from build123d import *

# Parameters (mm, degrees)
ESQUISSE1_R             = 1.7
BOSS_EXTRU_1_DEPTH      = 3
ENL_V_MAT_EXTRU_1_DEPTH = 25.197605652
CONG_1_R                = 3
CONG_2_R                = 3


with BuildPart() as part:
    # Esquisse1 → Boss.-Extru.1 (new body)
    with BuildSketch(Plane.XY):
        Polygon((12.594874651, 9.115771584), (-7.904447763, 6.416984589), (-2.628489378, 17.375533229), (16.571510622, 17.375533229), align=None)
        with Locations((8.467987162, 12.175533229)):
            Circle(ESQUISSE1_R, mode=Mode.SUBTRACT)
        with Locations((0.467987162, 12.175533229)):
            Circle(ESQUISSE1_R, mode=Mode.SUBTRACT)
    extrude(amount=BOSS_EXTRU_1_DEPTH)

    # Esquisse2 → Enlèv. mat.-Extru.1 (cut, through all)
    with BuildSketch(Plane.XY.offset(3)):
        with BuildLine():
            ThreePointArc((6.767987162, 12.175533229), (6.714089789, 12.99784824), (6.553319868, 13.806093213))
            ThreePointArc((6.553319868, 13.806093213), (7.755401396, 15.888159494), (9.837467677, 14.686077966))
            ThreePointArc((9.837467677, 14.686077966), (10.085002318, 13.441637293), (10.167987162, 12.175533229))
            ThreePointArc((10.167987162, 12.175533229), (8.467987162, 10.475533229), (6.767987162, 12.175533229))
        make_face()
    extrude(amount=-ENL_V_MAT_EXTRU_1_DEPTH, mode=Mode.SUBTRACT)

    # Congé1
    cong_1_edges = [part.edges().sort_by_distance(p)[0] for p in [
        (-2.628489378, 17.375533229, 1.5),
        (16.571510622, 17.375533229, 1.5),
        (12.594874651, 9.115771584, 1.5),
        (-7.904447763, 6.416984589, 1.5),
    ]]
    fillet(cong_1_edges, radius=CONG_1_R)

    # Congé2
    # the kernel refuses this fillet: 3 mm, written as the material it takes off along each edge
    with BuildSketch(Plane(origin=(-8.243247375, 17.375533229, 0), x_dir=(0, -1, 0), z_dir=(1, 0, 0))) as cong_2_piece_1:
        with BuildLine():
            CenterArc((CONG_2_R, -CONG_2_R), CONG_2_R, 90, 90)
            Line((0, -CONG_2_R), (0, 0))
            Line((0, 0), (CONG_2_R, 0))
        make_face()
    extrude(amount=27.54083508, mode=Mode.SUBTRACT)


solid = part.part
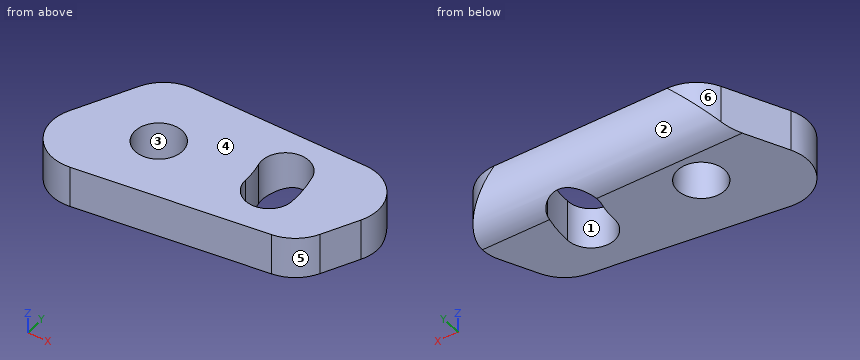
Work out the finished part from the listing and answer in its coordinate system (mm). Face numbers are marked on the shaded views. A direction names the side the tool comes from. Round coordinates to 2 decimals unless told otherwise and drop trailing zeros. Write each loop counter-clockwise with the first axis right and the second up, starting at its lowest first coordinate (ties: lowest second). Pieces come first, ordered by that corner, then holes. Notation, with made-up numbers: (72.25, 17) -> (92.25, 17) arc R22 ccw to (92.25, 38) -> close; hole circle Ø1 at (89, 6). An arc over 180 degrees is marked (long way). Write each question's results on one line, items separated by ' | '.
Item 1: A cutting plane is placed at A-A, the plane y = 15.25. Determine the outline of the cut face in (x, z), plus the area to 3 significant figures.
Result set:
outline: (-3.65, 0.13) -> (6.82, 0.13) -> (6.82, 3) -> (-3.65, 3) -> close; (9.57, 0.13) -> (14.67, 0.13) -> (14.67, 3) -> (9.57, 3) -> close | area: 44.7 mm^2
Item 2: Which of the six approach directions +Z, -Z, +X, -X, +Y, -Y give full straight-line access (tool end or side, diameter ignored) to the marked faces 1 and 2?
Result set:
face 1: +Z, -Z | face 2: -Z, +X, -X, +Y
Item 3: Find the intervals of material crossed by line 1 along X through (y, z) = (12, 1.8); line 2 along X through (y, z) = (13.5, 2.8); line 3 along Y through (x, z) = (0.5, 1.55), in increasing order. Write a range as [from, to].
Result set:
line 1: [-5.22, -1.22], [2.16, 6.78], [10.16, 13.98] | line 2: [-4.49, -0.6], [1.53, 6.63], [10.08, 14.67] | line 3: [7.52, 10.48], [13.88, 17]
Item 4: A cutting plane is placed at C-C, the plane z = 2.15. Determine the outline of the cut face in (x, y), plus the area to 3 significant figures.
Result set:
outline: (-5.5, 11.42) arc R3 ccw to (-2.4, 7.14) -> (10.99, 8.9) arc R3 ccw to (13.3, 10.58) -> (14.5, 13.07) arc R3 ccw to (12.65, 17.25) -> (-1.59, 17.25) arc R3 ccw to (-3.45, 15.68) -> close; hole circle Ø3.4 at (0.47, 12.18); hole (6.55, 13.81) arc R6.3 cw to (6.77, 12.18) arc R1.7 ccw to (10.17, 12.18) arc R9.7 ccw to (9.84, 14.69) arc R1.7 ccw to start | area: 144 mm^2
Item 5: A cutting plane is placed at D-D, the plane y = 13.5. Determine the outline of the cut face in (x, z).
Result set:
outline: (-4.49, 0) -> (-0.6, 0) -> (-0.6, 3) -> (-4.49, 3) -> close; (1.53, 0) -> (6.63, 0) -> (6.63, 3) -> (1.53, 3) -> close; (10.08, 0) -> (14.67, 0) -> (14.67, 3) -> (10.08, 3) -> close
Item 6: The mould has two halves that part along X. Classify the marked faces 3, 4, 5 and 6: +X half, -X half, draft (parallel to the pull), parting line (faces both ways), or undercut.
Result set:
face 3: undercut | face 4: draft | face 5: +X half | face 6: -X half
Item 7: A cutting plane is placed at B-B, the plane x = 9.5. Determine the outline of the cut face in (y, z).
Result set:
outline: (8.71, 0) -> (10.82, 0) -> (10.82, 3) -> (8.71, 3) -> close; (15.34, 0.16) arc R3 ccw to (17.38, 3) -> (15.34, 3) -> close
Item 8: A flat-ended cylindrical pin translates along its axis: P1, Ø3, axis at x = 0.47, y = 12.18, coming from the +Z side. Find the tip coordinate at first contact, or state that the pin passes through.
Result set:
P1: through
